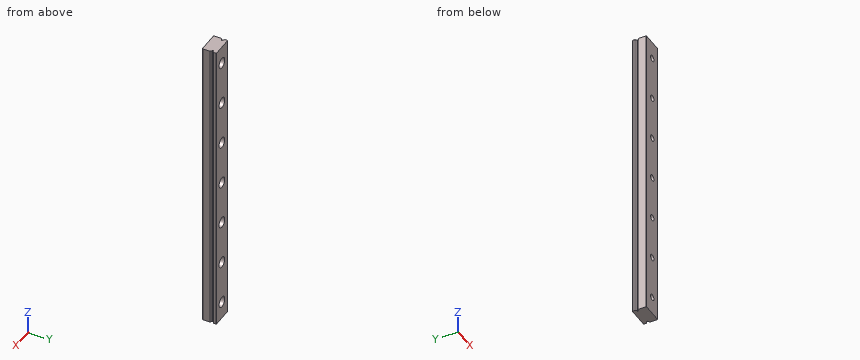
```python
from build123d import *

# Parameters (mm, degrees)
EXTRUDE_1_DEPTH        = 170
SKETCH_2_R             = 3
SKETCH_2_R_2           = 1.75
CUT_EXTRUDE_1_DEPTH    = 4.5
SKETCH_2_2_R           = 1.75
CUT_EXTRUDE_2_DEPTH    = 171.293863659
PATTERN_LINEAR_1_COUNT = 12
PATTERN_LINEAR_1_PITCH = 25


with BuildPart() as part:
    # Sketch 1 → Extrude 1 (new body)
    with BuildSketch(Plane.XY):
        with BuildLine():
            Line((-6, 3.7), (-5.7, 4))
            Line((-5.7, 4), (5.7, 4))
            Line((5.7, 4), (6, 3.7))
            Line((6, 3.7), (6, 2.449776022))
            ThreePointArc((6, 2.449776022), (5.561887715, 2.168810579), (5.297911886, 1.720256551))
            Line((5.297911886, 1.720256551), (4.687472904, 1.720256551))
            Line((4.687472904, 1.720256551), (4.687472904, 1.082255421))
            Line((4.687472904, 1.082255421), (5.292171789, 1.082255421))
            ThreePointArc((5.292171789, 1.082255421), (5.554928022, 0.621665058), (6, 0.333402583))
            Line((6, 0.333402583), (6, -3.7))
            Line((6, -3.7), (5.7, -4))
            Line((5.7, -4), (-5.7, -4))
            Line((-5.7, -4), (-6, -3.7))
            Line((-6, -3.7), (-6, 0.333402583))
            ThreePointArc((-6, 0.333402583), (-5.554928022, 0.621665058), (-5.292171789, 1.082255421))
            Line((-5.292171789, 1.082255421), (-4.687472904, 1.082255421))
            Line((-4.687472904, 1.082255421), (-4.687472904, 1.720256551))
            Line((-4.687472904, 1.720256551), (-5.297911886, 1.720256551))
            ThreePointArc((-5.297911886, 1.720256551), (-5.561887715, 2.168810579), (-6, 2.449776022))
            Line((-6, 2.449776022), (-6, 3.7))
        make_face()
    extrude(amount=EXTRUDE_1_DEPTH)

    # Sketch 2 → Cut-Extrude 1 (cut)
    with BuildSketch(Plane(origin=(0, 4, 0), x_dir=(1, 0, 0), z_dir=(0, 1, 0))):
        with Locations(Location((0.188190244, -10, 0), (0, 0, 270))):
            Circle(SKETCH_2_R)
        with Locations(Location((0.188190244, -10, 0), (0, 0, 270))):
            Circle(SKETCH_2_R_2, mode=Mode.SUBTRACT)
    cut_extrude_1 = extrude(amount=-CUT_EXTRUDE_1_DEPTH, mode=Mode.SUBTRACT)

    # Sketch 2_2 → Cut-Extrude 2 (cut, through all)
    with BuildSketch(Plane(origin=(0, 4, 0), x_dir=(1, 0, 0), z_dir=(0, 1, 0))):
        with Locations(Location((0.188190244, -10, 0), (0, 0, 270))):
            Circle(SKETCH_2_2_R)
    cut_extrude_2 = extrude(amount=-CUT_EXTRUDE_2_DEPTH, mode=Mode.SUBTRACT)

    # Pattern Linear 1: Cut-Extrude 1, Cut-Extrude 2 ×12
    with Locations(*[(0, 0, i * PATTERN_LINEAR_1_PITCH) for i in range(1, PATTERN_LINEAR_1_COUNT)]):
        add(cut_extrude_1, mode=Mode.SUBTRACT)
        add(cut_extrude_2, mode=Mode.SUBTRACT)


solid = part.part
```
Verification items for the finished model (mm, model axes). Round coordinates to 2 decimals unless told otherwise and drop trailing zeros. Order: outer loops, then holes, each group sorted by start corner. A loop starts at its lowest first (then second) coordinate and runs counter-clockwise, first axis right, second up. Notation, with made-up numbers: (-32.75, -24) - (-11.75, -24) arc R22 ccw to (-11.75, 12) - close; hole circle Ø11 at (32, 16.25). An arc over 180 degrees is marked (long way). Use CSV: the item, a comma, the result in double quotes.
(1) Thickness scan on probe 1 along X at (y, z) = (1.35, 10); probe 2 along Y at (x, z) = (4.75, 67); probe 3 along X at (y, z) = (1.5, 34.5). Record the ranges inside material, lowest first. Write a range as from..to.
Entries:
probe 1,"-4.69..-2.81, 3.19..4.69"
probe 2,"-4..1.08, 1.72..4"
probe 3,"-4.69..-2.77, 3.15..4.69"
(2) Section check A-A on z = 60. Record the boundary of the cut face in (x, y), and give its area (3 significant figures).
Entries:
outline,"(-6, -3.7) - (-5.7, -4) - (-1.56, -4) - (-1.56, -0.5) - (-2.81, -0.5) - (-2.81, 4) - (-5.7, 4) - (-6, 3.7) - (-6, 2.45) arc R1.12 cw to (-5.3, 1.72) - (-4.69, 1.72) - (-4.69, 1.08) - (-5.29, 1.08) arc R1.12 cw to (-6, 0.33) - close; (1.94, -4) - (5.7, -4) - (6, -3.7) - (6, 0.33) arc R1.12 cw to (5.29, 1.08) - (4.69, 1.08) - (4.69, 1.72) - (5.3, 1.72) arc R1.12 cw to (6, 2.45) - (6, 3.7) - (5.7, 4) - (3.19, 4) - (3.19, -0.5) - (1.94, -0.5) - close"
area,"53.5 mm^2"
(3) Section check B-B on z = 42.5. Record the boundary of the cut face in (x, y), and give its area (3 significant figures).
Entries:
outline,"(-6, -3.7) - (-5.7, -4) - (5.7, -4) - (6, -3.7) - (6, 0.33) arc R1.12 cw to (5.29, 1.08) - (4.69, 1.08) - (4.69, 1.72) - (5.3, 1.72) arc R1.12 cw to (6, 2.45) - (6, 3.7) - (5.7, 4) - (-5.7, 4) - (-6, 3.7) - (-6, 2.45) arc R1.12 cw to (-5.3, 1.72) - (-4.69, 1.72) - (-4.69, 1.08) - (-5.29, 1.08) arc R1.12 cw to (-6, 0.33) - close"
area,"92.8 mm^2"
(4) Section check C-C on y = -2. Record the boundary of the cut face in (x, z).
Entries:
outline,"(-6, 0) - (6, 0) - (6, 170) - (-6, 170) - close; hole circle Ø3.5 at (0.19, 10); hole circle Ø3.5 at (0.19, 35); hole circle Ø3.5 at (0.19, 60); hole circle Ø3.5 at (0.19, 85); hole circle Ø3.5 at (0.19, 110); hole circle Ø3.5 at (0.19, 135); hole circle Ø3.5 at (0.19, 160)"
(5) Gauge pin test, flat end, axial feed: pin 1 Ø1.8 at (x, z) = (0.5, 160.5) entering from +Y. Record the tip position at first contact, or that the pin passes through.
Entries:
pin 1,"through"
